The listing builds one solid part. Answer for the finished solid, in the listing's coordinates (mm). A direction names the side the tool comes from. Give positions to 0.01 mm unless a question says otherwise; leave off trailing zeros. Order: outer loops, then holes, each group sorted by start corner. A loop starts at its lowest first (then second) coordinate and runs counter-clockwise, first axis right, second up. Notation, with made-up numbers: (-30.5, 41.25) - (-17.5, 41.25) arc R22 cw to (-17.5, 69.25) - close; hole circle Ø5 at (8, -28.75). An arc over 180 degrees is marked (long way). Answer in a Markdown table with one row per item.
from build123d import *

# Parameters (mm, degrees)
F0_R     = 3.175
F0_R_2   = 1.5875
F1_DEPTH = 3.048


with BuildPart() as f1:
    # F0 (on Front) → F1 (new body)
    with BuildSketch(Plane.XZ):
        with BuildLine():
            Line((-39.872363, 5.642511), (-40.393674, 1.391583))
            ThreePointArc((-40.393674, 1.391583), (-25.329494, -14.251993), (-8.750471, -0.223914))
            ThreePointArc((-8.750471, -0.223914), (-8.671445, 0.687703), (-8.645073, 1.602358))
            ThreePointArc((-8.645073, 1.602358), (-8.676443, 2.599858), (-8.770428, 3.593415))
            ThreePointArc((-8.770428, 3.593415), (-23.476439, 17.443016), (-39.872363, 5.642511))
        make_face()
        with Locations((-24.520073, 1.602358)):
            Circle(F0_R, mode=Mode.SUBTRACT)
        with BuildLine():
            ThreePointArc((-39.872363, 5.642511), (-40.277029, 3.534708), (-40.393674, 1.391583))
            Line((-40.393674, 1.391583), (-39.872363, 5.642511))
        make_face()
        with BuildLine():
            ThreePointArc((-8.750471, -0.223914), (-25.329494, -14.251993), (-40.393674, 1.391583))
            Line((-40.393674, 1.391583), (-40.375196, 0))
            Line((-40.375196, 0), (-33.078623, -62.887975))
            ThreePointArc((-33.078623, -62.887975), (-25.039092, -53.319184), (-15.950314, -61.897642))
            ThreePointArc((-15.950314, -61.897642), (-18.378295, -67.883554), (-24.290135, -70.486702))
            Line((-24.290135, -70.486702), (20.023751, -69.834282))
            ThreePointArc((20.023751, -69.834282), (11.969402, -61.897642), (20.023751, -53.961002))
            Line((20.023751, -53.961002), (-6.122254, -53.576062))
            ThreePointArc((-6.122254, -53.576062), (-11.980182, -50.87129), (-13.902635, -44.712127))
            Line((-13.902635, -44.712127), (-8.750471, -0.223914))
        make_face()
        with BuildLine():
            Line((-33.995798, 53.561768), (-39.872363, 5.642511))
            ThreePointArc((-39.872363, 5.642511), (-23.476439, 17.443016), (-8.770428, 3.593415))
            Line((-8.770428, 3.593415), (-15.091838, 53.596992))
            ThreePointArc((-15.091838, 53.596992), (-15.035447, 53.000858), (-15.016625, 52.402358))
            ThreePointArc((-15.016625, 52.402358), (-25.12241, 42.895081), (-33.995798, 53.561768))
        make_face()
        with Locations((-30.164933, 36.977328)):
            Circle(F0_R_2, mode=Mode.SUBTRACT)
        with BuildLine():
            ThreePointArc((-15.091838, 53.596992), (-24.559373, 61.927342), (-33.995798, 53.561768))
            ThreePointArc((-33.995798, 53.561768), (-25.12241, 42.895081), (-15.016625, 52.402358))
            ThreePointArc((-15.016625, 52.402358), (-15.035447, 53.000858), (-15.091838, 53.596992))
        make_face()
        with Locations((-24.541625, 52.402358)):
            Circle(F0_R, mode=Mode.SUBTRACT)
        with BuildLine():
            ThreePointArc((-15.950314, -61.897642), (-25.039092, -53.319184), (-33.078623, -62.887975))
            ThreePointArc((-33.078623, -62.887975), (-30.258263, -68.314248), (-24.543098, -70.490426))
            Line((-24.543098, -70.490426), (-24.290135, -70.486702))
            ThreePointArc((-24.290135, -70.486702), (-18.378295, -67.883554), (-15.950314, -61.897642))
        make_face()
        with Locations((-24.543098, -61.897642)):
            Circle(F0_R, mode=Mode.SUBTRACT)
        with BuildLine():
            Line((-24.290135, -70.486702), (-24.543098, -70.490426))
            ThreePointArc((-24.543098, -70.490426), (-24.416603, -70.489495), (-24.290135, -70.486702))
        make_face()
        with BuildLine():
            ThreePointArc((27.844402, -61.897642), (25.560723, -56.326447), (20.023751, -53.961002))
            ThreePointArc((20.023751, -53.961002), (11.969402, -61.897642), (20.023751, -69.834282))
            ThreePointArc((20.023751, -69.834282), (25.560723, -67.468837), (27.844402, -61.897642))
        make_face()
        with Locations((19.906902, -61.897642)):
            Circle(F0_R, mode=Mode.SUBTRACT)
    extrude(amount=F1_DEPTH)


solid = f1.part
Item 1: Determine the mould class of faces 1 (the face through (-22, -3.048, -18)), 2 (the face through (-28.7, -1.5, 36.37)), 3 (the face through (-24.366, -1.503, 61.926)) for opening direction Z: pulls with the +Z half, pulls with the -Z half, needs draft (parallel to the pull), parting line crosses it, or undercut.
Answer block:
| item | result |
|---|---|
| face 1 | needs draft |
| face 2 | undercut |
| face 3 | pulls with the +Z half |
Item 2: Find section C-C on z = 13. Write down the section's boundary in (x, y), then the cut area to 3 significant figures.
Answer block:
| item | result |
|---|---|
| outline | (-38.97, -3.05) - (-9.96, -3.05) - (-9.96, 0) - (-38.97, 0) - close |
| area | 88.4 mm² |
Item 3: Find section D-D on x = 14.5. Write down the section's boundary in (y, z).
Answer block:
| item | result |
|---|---|
| outline | (-3.05, -69.92) - (0, -69.92) - (0, -53.88) - (-3.05, -53.88) - close |
Item 4: Find section A-A on x = -12. Write down the section's boundary in (y, z).
Answer block:
| item | result |
|---|---|
| outline | (-3.05, -70.31) - (0, -70.31) - (0, -50.85) - (-3.05, -50.85) - close; (-3.05, -28.28) - (0, -28.28) - (0, 29.14) - (-3.05, 29.14) - close |
Item 5: Find section B-B on y = -2. Count the separate pieces of the cut face and the enclosed holes in it, then the cut area to 3 significant figures.
Answer block:
| item | result |
|---|---|
| separate pieces | 1 |
| enclosed holes | 5 |
| area | 3,700 mm² |
Item 6: Which of the six approach directions +Z, -Z, +X, -X, +Y, -Y give full straight-line access (tool end or side, diameter ignored) to faces 4 (the face through (-22, 0, -18)), 5 (the face through (-11.363, -1.503, -22.779))?
Answer block:
| item | result |
|---|---|
| face 4 | +Z, -Z, +X, -X, +Y |
| face 5 | +X, +Y, -Y |
Item 7: Each of these flat-tipped pins is pushed along its axis until it touches: P1, Ø5.5, axis at x = -24.54, z = -61.9, coming from the +Y side; P2, Ø1.5, axis at y = -2.5, z = -6, coming from the +X side. Where does it stop, or does it pass through?
Answer block:
| item | result |
|---|---|
| P1 | through |
| P2 | x = -9.33 |
Item 8: Consider line 1 (X direction, y = -1.2, z = -63.5); line 2 (Z direction, x = 18, y = -0.3); line 3 (Z direction, x = 20, y = -2.9). Determine where each line is inside the solid, lowest interval first.
Answer block:
| item | result |
|---|---|
| line 1 | -32.99 to -27.28, -21.8 to 17.17, 22.65 to 27.68 |
| line 2 | -69.86 to -64.44, -59.36 to -53.93 |
| line 3 | -69.83 to -65.07, -58.72 to -53.96 |
